The listing builds one solid part. Answer for the finished solid, in the listing's coordinates (mm). Round coordinates to 2 decimals unless told otherwise and drop trailing zeros. Write each loop counter-clockwise with the first axis right and the second up, starting at its lowest first coordinate (ties: lowest second). Pieces come first, ordered by that corner, then holes. Notation, with made-up numbers: M 58,-36.75 L 105,-36.75 A17 ccw 105,-9.75 Z; hole C -33.5,-12.5 d1. An arc over 180 degrees is marked long. Write each question's results on one line, items separated by ' | '.
Autodesk Inventor part; units mm, degrees
ref_plane "YZ Plane" through (0, 0, 0) normal (1, 0, 0) x (0, 1, 0)
ref_plane "XZ Plane" through (0, 0, 0) normal (0, 1, 0) x (-1, 0, 0)
ref_plane "XY Plane" through (0, 0, 0) normal (0, 0, 1) x (1, 0, 0)
sketch "Sketch1" plane through (0, 0, 0) normal (1, 0, 0) x (0, 1, 0)
  line L0 (50.8, 190.5) -> (0, 190.5)
  line L1 (0, 190.5) -> (0, 0)
  line L2 (0, 0) -> (50.8, 0)
  line L3 (50.8, 0) -> (50.8, 190.5)
  line L4 (0, 196.85) -> (50.8, 190.5)
  line L5 (0, 196.85) -> (0, 190.5)
  line L6 (0, 0) -> (50.8, 0)
  line L7 (0, 0) -> (0, 0)
  line L8 (50.8, 0) -> (0, 0)
  line L9 (0, 0) -> (0, 0)
  line L10 (0, -6.35) -> (50.8, 0)
  line L11 (0, -6.35) -> (0, 0)
  line L12 (0, 0) -> (76.2, 0)
  line L13 (76.2, 0) -> (76.2, 190.5)
  line L14 (76.2, 190.5) -> (0, 196.85)
  line L15 (76.2, 0) -> (0, -6.35)
  dimension "d0" = 76.2
extrude "Extrusion1" add sketch "Sketch1" along normal blind 2.54
hole "Hole1" at (2.54, 63.5, 178.8143) direction (-1, 0, 0) diameter 6.35 end through all
pattern_linear "Rectangular Pattern1" count 2 spacing 152.4 along (0, 0, -1) of "Hole1"
properties part number "mountPiece"
1) The mould has two halves that part along Y. Classify faces 1 (the face through (1.25, 60.82, 24.71)), 2 (the face through (2.54, 38, 97)), 3 (the face through (1.25, 38.63, -3.13)): +Y half, -Y half, draft (parallel to the pull), parting line (faces both ways), or undercut.
Return value:
face 1: undercut | face 2: draft | face 3: +Y half
2) Section C-C (y = 33) is taken. Determine the outline of the cut face in (x, z).
Return value:
outline: M 0,-3.6 L 2.54,-3.6 L 2.54,194.1 L 0,194.1 Z
3) Section B-B (y = 63.5) is taken. Determine the outline of the cut face in (x, z), then the cut area to 3 significant figures.
Return value:
outline: M 0,-1.06 L 2.54,-1.06 L 2.54,23.24 L 0,23.24 Z; M 0,29.59 L 2.54,29.59 L 2.54,175.64 L 0,175.64 Z; M 0,181.99 L 2.54,181.99 L 2.54,191.56 L 0,191.56 Z | area: 457 mm²
4) Each of these flat-tipped pins is pushed along its axis until it touches: pin 1 (1 mm diameter, centred on x = 2, y = 57.5, fed in from -Z); pin 2 (5.5 mm diameter, centred on y = 63.5, z = 26.41, fed in from -X). Where does it stop, or does it pass through?
Return value:
pin 1: z = -1.6 | pin 2: through
5) Section A-A (x = 1.35) is taken. Determine the outline of the cut face in (y, z) (3 decimals), then the cut area to 3 significant figures.
Return value:
outline: M 0,-6.35 L 76.2,0 L 76.2,190.5 L 0,196.85 Z; hole C 63.5,26.414 d6.35; hole C 63.5,178.814 d6.35 | area: 14,900 mm²
6) Find the intervals of material crossed by line 1 (Z direction, x = 0.6, y = 63.5); line 2 (Y direction, x = 1.25, z = 180); line 3 (Z direction, x = 1.6, y = 65), in increasing order.
Return value:
line 1: -1.06 to 23.24, 29.59 to 175.64, 181.99 to 191.56 | line 2: 0 to 60.55, 66.45 to 76.2 | line 3: -0.93 to 23.62, 29.21 to 176.02, 181.61 to 191.43
